Check sheet for the modelled part. Datum: model origin and axes. Units: mm. Coordinates: 2 decimals unless noted, no trailing zeros. Loops run counter-clockwise (first coordinate to the right, second up) from the corner with the lowest first, then second, coordinate; pieces in that order, holes last. Notation, with made-up numbers: M -4,72.25 L 40,72.25 A19 cw 40,85.25 Z; hole C 1,10 d1. An arc over 180 degrees is marked long. Use CSV: the item, a comma, the result in double quotes. Start each with the question number.
(1) Section check A-A on x = -85. Record the cut outline in (y, z), and give its area (3 significant figures).
(2) Go/stop test with flat-tipped pins: pin 1 Ø2.5 at (x, y) = (-12.5, -15.5) entering from +Z; pin 2 Ø4 at (x, z) = (-477.5, 71.5) entering from +Y; pin 3 Ø20 at (x, y) = (1255, 9.5) entering from +Z. Record where each tip stops, or that it passes through.
(3) Scan lines: line 1 (Y direction, x = 289.5, z = -52.5); line 2 (X direction, y = 14, z = 60.5); line 3 (Z direction, x = -800.5, y = -12.5). Record each from-to range of solid material in increasing order.
from build123d import *

# Parameters (mm, degrees)
F1_W     = 40
F1_H     = 33
F3_DEPTH = 1275
F2_W     = 80
F2_H     = 100
F4_DEPTH = 25


with BuildPart() as f3:
    # F1 (on Right) → F3 (new body, symmetric)
    with BuildSketch(Plane.YZ):
        Polygon((20, 33), (20, 63), (17, 66), (12, 66), (12, 80), (4, 80), (4, 66), (-4, 66), (-4, 80), (-12, 80), (-12, 66), (-17, 66), (-20, 63), (-20, 33), align=None)
        with Locations((0, 16.5)):
            Rectangle(F1_W, F1_H)
        with Locations((0, -16.5)):
            Rectangle(F1_W, F1_H)
        Polygon((20, -63), (20, -33), (-20, -33), (-20, -63), (-17, -66), (-12, -66), (-12, -52), (-4, -52), (-4, -66), (4, -66), (4, -52), (12, -52), (12, -66), (17, -66), align=None)
    extrude(amount=F3_DEPTH, both=True)

    # F2 (on Front) → F4 (cut, symmetric)
    with BuildSketch(Plane.XZ):
        with Locations((-1275, 83)):
            Rectangle(F2_W, F2_H)
        with Locations((-1275, -83)):
            Rectangle(F2_W, F2_H)
        with Locations((1275, 83)):
            Rectangle(F2_W, F2_H)
        with Locations((1275, -83)):
            Rectangle(F2_W, F2_H)
    extrude(amount=F4_DEPTH, both=True, mode=Mode.SUBTRACT)


solid = f3.part
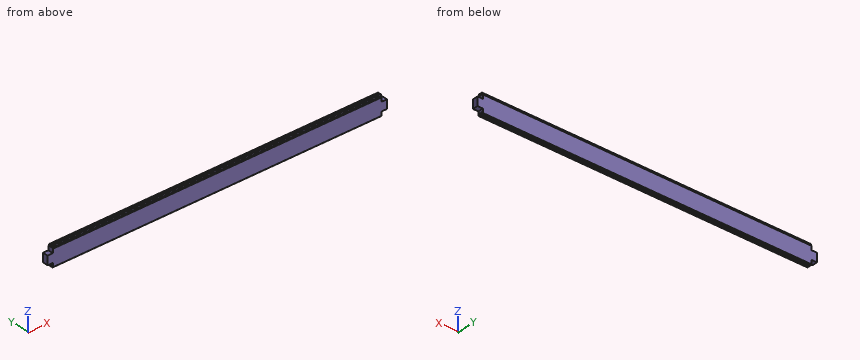
Outcome:
1,outline,"M -20,-63 L -17,-66 L -12,-66 L -12,-52 L -4,-52 L -4,-66 L 4,-66 L 4,-52 L 12,-52 L 12,-66 L 17,-66 L 20,-63 L 20,63 L 17,66 L 12,66 L 12,80 L 4,80 L 4,66 L -4,66 L -4,80 L -12,80 L -12,66 L -17,66 L -20,63 Z"
1,area,"5,260 mm²"
2,pin 1,"stops at z = 66"
2,pin 2,"stops at y = 12"
2,pin 3,"stops at z = 33"
3,line 1,"y = -20 to -12, -4 to 4, 12 to 20"
3,line 2,"x = -1235 to 1235"
3,line 3,"z = -66 to 66"
